Part print with two shaded views. Sizes in mm from the minimum x, y, z corner. A direction names the side the tool comes from. Coordinates: 2 decimals unless noted, no trailing zeros. Write each loop counter-clockwise with the first axis right and the second up, starting at its lowest first coordinate (ties: lowest second). Pieces come first, ordered by that corner, then holes. Notation, with made-up numbers: (73, -15.5) - (83, -15.5) arc R17 cw to (83, -5.5) - close; hole circle Ø3 at (29, 46). An arc over 180 degrees is marked (long way). Answer in a Markdown table with one row per item. Add a question column.
Q1. Band-saw the part on D-D (z = 39). List the corners of the cut face in (x, y), and give its area (3 significant figures).
Q2. Drill centre lines: line 1 along Z through (x, y) = (25, 22); line 2 along Z through (x, y) = (24, 27); line 3 along X through (y, z) = (28.5, 74.5). Where is each one in solid material? Low to high. Write a range as from..to.
Q3. Two-plate mould, pull along Z, no slides. Class the marked faces 4, 5 and 6: +Z half, -Z half, draft (parallel to the pull), parting line (faces both ways), or undercut.
Q4. 3-axis set-ups, long thin cutter, end or side, ignore diameter. For the marked faces 1, 2 and 3: which of +Z, -Z, +X, -X, +Y, -Y reach the whole face in a straight line?
Q5. Band-saw the part on B-B (y = 22.5). List the corners of the cut face in (x, z).
Q6. Band-saw the part on C-C (x = 22.5). List the corners of the cut face in (y, z), and give its area (3 significant figures).
Q7. Band-saw the part on A-A (z = 60). List the corners of the cut face in (x, y).
Q8. Pin check, flat tips, straight feed: pin 1 (10 mm diameter, centred on x = 15, z = 41, fed in from -Y); pin 2 (9 mm diameter, centred on y = 22.5, z = 60, fed in from -X); pin 3 (4 mm diameter, centred on x = 25.5, z = 72, fed in from +Y); pin 4 (3 mm diameter, centred on x = 38, y = 29, fed in from +Z). Stop position of each tip, or through.
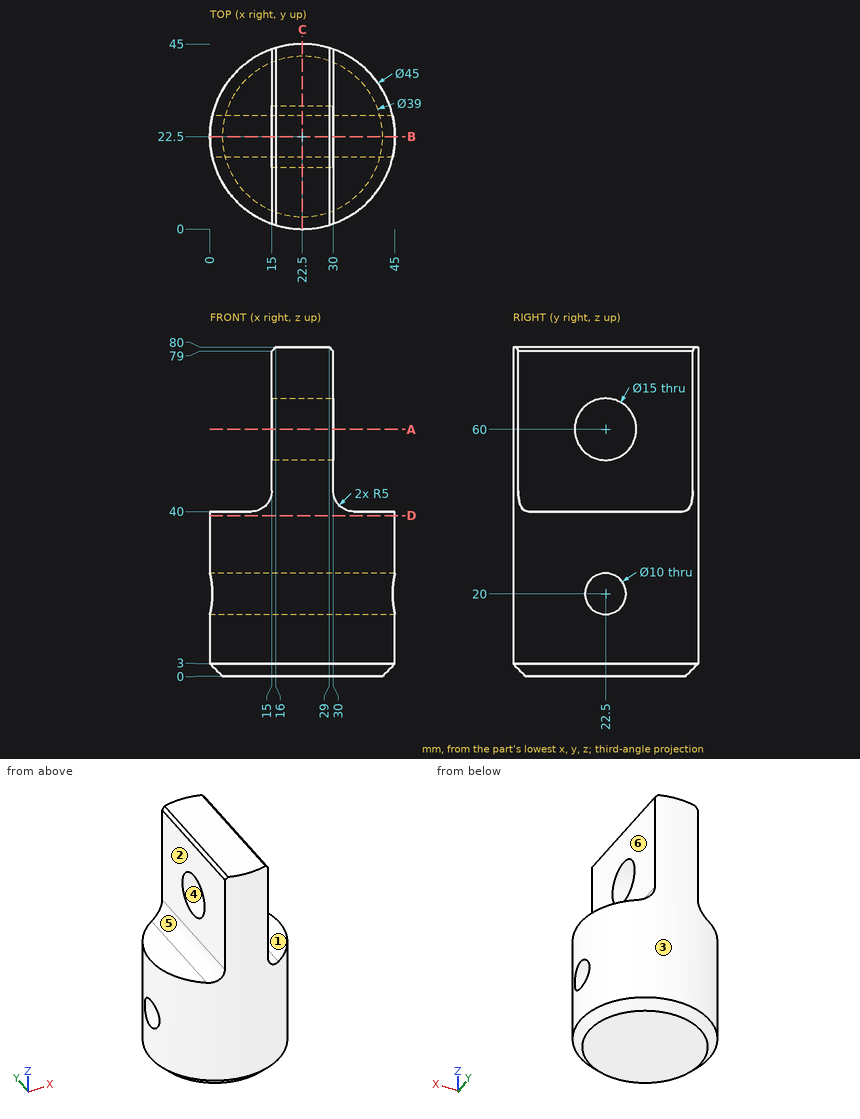
Checked values:
| question | item | result |
|---|---|---|
| 1 | outline | circle Ø45 at (22.5, 22.5) |
| 1 | area | 1,590 mm² |
| 2 | line 1 | z = 0..15.03, 24.97..52.52, 67.48..80 |
| 2 | line 2 | z = 0..17.82, 22.18..54, 66..80 |
| 2 | line 3 | x = 15..30 |
| 3 | face 4 | undercut |
| 3 | face 5 | +Z half |
| 3 | face 6 | draft |
| 4 | face 1 | +Z, +X, +Y, -Y |
| 4 | face 2 | +Z, -X, +Y, -Y |
| 4 | face 3 | +Z, -Z |
| 5 | outline | (0, 3) - (3, 0) - (42, 0) - (45, 3) - (45, 15) - (0, 15) - close; (0, 25) - (45, 25) - (45, 40) - (35, 40) arc R5 cw to (30, 45) - (30, 52.5) - (15, 52.5) - (15, 45) arc R5 cw to (10, 40) - (0, 40) - close; (15, 67.5) - (30, 67.5) - (30, 79) - (29, 80) - (16, 80) - (15, 79) - close |
| 6 | outline | (0, 3) - (3, 0) - (42, 0) - (45, 3) - (45, 80) - (0, 80) - close; hole circle Ø15 at (22.5, 60); hole circle Ø10 at (22.5, 20) |
| 6 | area | 3,340 mm² |
| 7 | outline | (15, 1.29) arc R22.5 ccw to (30, 1.29) - (30, 15) - (15, 15) - close; (15, 30) - (30, 30) - (30, 43.71) arc R22.5 ccw to (15, 43.71) - close |
| 8 | pin 1 | stops at y = 0.14 |
| 8 | pin 2 | passes through |
| 8 | pin 3 | stops at y = 44.98 |
| 8 | pin 4 | stops at z = 40 |
